The listing builds one solid part. Answer for the finished solid, in the listing's coordinates (mm). A direction names the side the tool comes from. Give positions to 0.01 mm unless a question says otherwise; leave off trailing zeros. Order: outer loops, then holes, each group sorted by start corner. A loop starts at its lowest first (then second) coordinate and runs counter-clockwise, first axis right, second up. Notation, with made-up numbers: (77.25, -12.5) - (96.25, -12.5) arc R16 ccw to (96.25, 4.5) - close; hole circle Ø3 at (46, 43). An arc over 180 degrees is marked (long way). Write each question's results on one line, items separated by ' | '. Start each with the question number.
1. Section B-B (y = 24) is taken. Give the vertices of the cut face in (x, z).
2. Section C-C (x = -42) is taken. Give the vertices of the cut face in (y, z).
3. Section A-A (z = 0) is taken. Give the vertices of the cut face in (x, y) (3 decimals), and give its area (3 significant figures).
4. Determine the mould class of faces 1 (the face through (-59, 20, 0)), 2 (the face through (-58, 33, 4)), 3 (the face through (-16.644, 1.521, -0.451)) for opening direction X: released by +X, released by -X, zero draft, split by the parting line, or undercut.
5. Which of the six approach directions +Z, -Z, +X, -X, +Y, -Y give full straight-line access (tool end or side, diameter ignored) to faces 4 (the face through (-34, 3, 0)), 5 (the face through (-58, 34, 3)), 6 (the face through (-58, 34, -3))?
6. Flat-ended cylindrical pins translate along their axes: pin 1 (3.5 mm diameter, centred on x = -57, y = 34, fed in from -Z); pin 2 (1 mm diameter, centred on y = 23, z = 3.5, fed in from +X); pin 3 (5 mm diameter, centred on x = -37.925, z = 0, fed in from +Y); pin 4 (1 mm diameter, centred on x = -57, z = -4, fed in from +Y). Find the tip coordinate at first contact, or state that the pin passes through.
7. Find the intervals of material crossed by L1, parallel to X at y = 2.4, z = 0 (3 decimals); L2, parallel to X at y = 6, z = 0.25; L3, parallel to Y at x = -48, z = 2.25, in increasing order.
from build123d import *

# Parameters (mm, degrees)
BOSS_EXTRUDE2_DEPTH = 5
SKETCH8_R           = 1.5
CUT_EXTRUDE3_DEPTH  = 3
FILLET7_R           = 5
FILLET8_R           = 2.5
SKETCH9_W           = 13.075
SKETCH9_H           = 10
CUT_EXTRUDE4_DEPTH  = 3
SKETCH11_W          = 3
SKETCH11_H          = 6
BOSS_EXTRUDE4_DEPTH = 3


with BuildPart() as part:
    # Sketch5 → Boss-Extrude2 (new body, symmetric)
    with BuildSketch(Plane.XY):
        Polygon((0, 3), (0, 0), (-59, 0), (-59, 33), (-56, 33), (-56, 3), align=None)
    extrude(amount=BOSS_EXTRUDE2_DEPTH, both=True)

    # Sketch8 → Cut-Extrude3 (cut)
    with BuildSketch(Plane(origin=(0, 3, 0), x_dir=(1, 0, 0), z_dir=(0, 1, 0))):
        with Locations((-18.075, 0)):
            Circle(SKETCH8_R)
        with Locations((-37.925, 0)):
            Circle(SKETCH8_R)
    extrude(amount=-CUT_EXTRUDE3_DEPTH, mode=Mode.SUBTRACT)

    # Fillet7
    fillet7_edges = [part.edges().sort_by_distance(p)[0] for p in [
        (-59, 0, 0),
    ]]
    fillet(fillet7_edges, radius=FILLET7_R)

    # Fillet8
    fillet8_edges = [part.edges().sort_by_distance(p)[0] for p in [
        (-56, 3, 0),
    ]]
    fillet(fillet8_edges, radius=FILLET8_R)

    # Sketch9 → Cut-Extrude4 (cut)
    with BuildSketch(Plane(origin=(0, 3, 0), x_dir=(1, 0, 0), z_dir=(0, 1, 0))):
        with Locations((-6.5375, 0)):
            Rectangle(SKETCH9_W, SKETCH9_H)
    extrude(amount=-CUT_EXTRUDE4_DEPTH, mode=Mode.SUBTRACT)

    # Sketch11 → Boss-Extrude4 (add)
    with BuildSketch(Plane(origin=(0, 33, 0), x_dir=(1, 0, 0), z_dir=(0, 1, 0))):
        with Locations((-57.5, 0)):
            Rectangle(SKETCH11_W, SKETCH11_H)
    extrude(amount=BOSS_EXTRUDE4_DEPTH)


solid = part.part
Reported:
1) outline: (-59, -5) - (-56, -5) - (-56, 5) - (-59, 5) - close
2) outline: (0, -5) - (3, -5) - (3, 5) - (0, 5) - close
3) outline: (-59, 5) arc R5 ccw to (-54, 0) - (-39.425, 0) - (-39.425, 3) - (-53.5, 3) arc R2.5 cw to (-56, 5.5) - (-56, 36) - (-59, 36) - close; (-36.425, 0) - (-19.575, 0) - (-19.575, 3) - (-36.425, 3) - close; (-16.575, 0) - (-13.075, 0) - (-13.075, 3) - (-16.575, 3) - close | area: 215 mm²
4) face 1: released by -X | face 2: zero draft | face 3: undercut
5) face 4: +Z, -Z, +X, +Y | face 5: +Z, +X, -X, +Y | face 6: -Z, +X, -X, +Y
6) pin 1: z = -5 | pin 2: x = -56 | pin 3: y = 3 | pin 4: y = 33
7) L1: -58.271 to -39.425, -36.425 to -19.575, -16.575 to -13.075 | L2: -59 to -56 | L3: 0 to 3
